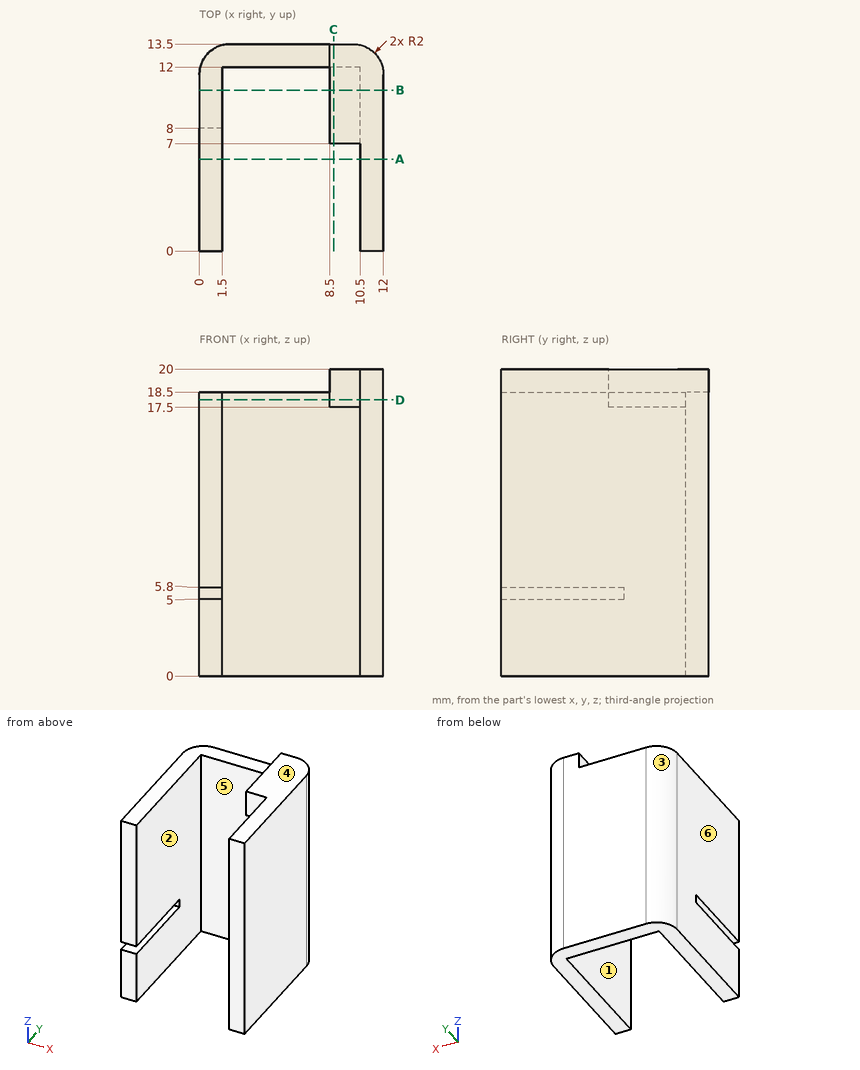
Study the drawing (mm; zero at the part's minimum x, y, z) and answer. A direction names the side the tool comes from. Coordinates: 2 decimals unless noted, no trailing zeros. Order: outer loops, then holes, each group sorted by start corner. A loop starts at its lowest first (then second) coordinate and runs counter-clockwise, first axis right, second up. Notation, with made-up numbers: M 60.25,-23.75 L 119.25,-23.75 A10 cw 119.25,-7.75 Z; hole C 41,60.5 d4. An arc over 180 degrees is marked long. Answer as a JSON object with one key per item and string values. Group by question number.
1. Section B-B on y = 10.5 is taken. Write down the section's boundary in (x, z), then the cut area to 4 significant figures.
2. Section D-D on z = 18 is taken. Write down the section's boundary in (x, y).
3. Section A-A on y = 6 is taken. Write down the section's boundary in (x, z), then the cut area to 4 significant figures.
4. A tool of negligible diameter and unlimited length cuts with its end or side. For the marked faces 1, 2 and 3, from which of +Z, -Z, +X, -X, +Y, -Y can it reach the whole face along a straight path? Write none if from no direction.
5. Straight lines are drawn through the part: line 1 (X direction, y = 10.25, z = 7.25); line 2 (Y direction, x = 5.5, z = 2.25); line 3 (Z direction, x = 1.25, y = 11.25). For each, find the intervals that lie inside material, in ascending order.
6. Section C-C on x = 8.75 is taken. Write down the section's boundary in (y, z).
7. Determine the mould class of the marked faces 4, 5 and 6 for opening direction X: released by +X, released by -X, zero draft, split by the parting line, or undercut.
8. Flat-ended cylindrical pins translate along their axes: P1, Ø0.8, axis at x = 0.5, y = 4.5, coming from the +Z side; P2, Ø1.6, axis at x = 9.5, z = 18.5, coming from the -Y side; P3, Ø7, axis at x = 6, z = 6.5, coming from the -Y side. Find the tip coordinate at first contact, or state that the pin passes through.
Values follow:
{
 "1": {"outline": "M 0,0 L 1.5,0 L 1.5,18.5 L 0,18.5 Z; M 8.5,17.5 L 10.5,17.5 L 10.5,0 L 12,0 L 12,20 L 8.5,20 Z", "area": "62.75 mm2"},
 "2": {"outline": "M 0,0 L 1.5,0 L 1.5,12 L 8.5,12 L 8.5,7 L 10.5,7 L 10.5,0 L 12,0 L 12,11.5 A2 ccw 10,13.5 L 2,13.5 A2 ccw 0,11.5 Z"},
 "3": {"outline": "M 0,0 L 1.5,0 L 1.5,5 L 0,5 Z; M 0,5.8 L 1.5,5.8 L 1.5,18.5 L 0,18.5 Z; M 10.5,0 L 12,0 L 12,20 L 10.5,20 Z", "area": "56.55 mm2"},
 "4": {"face 1": "-Z, -Y", "face 2": "+Z, -Z, -Y", "face 3": "+Z, -Z, -X, +Y"},
 "5": {"line 1": "0 to 1.5, 10.5 to 12", "line 2": "12 to 13.5", "line 3": "0 to 18.5"},
 "6": {"outline": "M 7,17.5 L 12,17.5 L 12,0 L 13.5,0 L 13.5,20 L 7,20 Z"},
 "7": {"face 4": "zero draft", "face 5": "undercut", "face 6": "released by -X"},
 "8": {"P1": "z = 18.5", "P2": "y = 7", "P3": "y = 12"}
}
